Autodesk Inventor part; units mm, degrees
ref_plane "YZ Plane" through (0, 0, 0) normal (1, 0, 0) x (0, 1, 0)
ref_plane "XZ Plane" through (0, 0, 0) normal (0, 1, 0) x (-1, 0, 0)
ref_plane "XY Plane" through (0, 0, 0) normal (0, 0, 1) x (1, 0, 0)
sketch "Sketch1" plane through (0, 0, 0) normal (0, 0, 1) x (1, 0, 0)
  circle A0 centre (0, 0) radius 0.8
  circle A1 centre (0, 0) radius 0.4
  circle A2 centre (0, 0) radius 0.8
  circle A3 centre (0, 0) radius 1.5
  line L0 (0, 0) -> (-1.5, 0)
  line L1 (-0.8, 0) -> (-1.5, 0)
  line L2 (-2.1, 5) -> (-0.9, 5)
  line L3 (-0.9, 5) -> (-0.9, -5)
  line L4 (-0.9, -5) -> (-2.1, -5)
  line L5 (-2.1, -5) -> (-2.1, 5)
  line L6 (-2.1, 5) -> (-0.9, -5) construction
  line L7 (-0.9, 5) -> (-2.1, -5) construction
  point P0 (-0.9, -1.2)
  point P1 (-0.9, 1.2)
  dimension "d0" = 1.6
  dimension "d1" = 3
  dimension "d2" = 1.2
  dimension "d3" = 10
extrude "Extrusion1" add sketch "Sketch1" against normal blind 20 contours L3 A3 | L3 A3 L0 | L0 A3 L3 | A3 L3 L4 L5 L2
fillet "Fillet1" radius 0.5 2 edges at (-0.9, -1.2, -10) (-0.9, 1.2, -10)
chamfer "Chamfer1" distance 0.3 angle 45 2 edges at (-0.8, 0, -20) (-0.8, 0, 0)
sketch "Sketch2" plane through (-0.9, 5, 0) normal (1, 0, 0) x (0, 0, -1)
  line L0 (20, -3.0404) -> (0, -3.0404)
  line L1 (20, 0) -> (20, -3.0404)
  line L2 (0, 0) -> (20, 0)
  line L3 (0, -3.0404) -> (0, 0)
  line L4 (20, 0) -> (20, -3.0404)
  line L5 (20, 0) -> (20, -1)
  line L6 (20, -1) -> (16, -1)
  line L7 (16, -1) -> (10, -1)
  line L8 (10, -1) -> (4, -1)
  line L9 (4, -1) -> (0, -1)
  line L10 (0, -3.0404) -> (0, 0)
  circle A0 centre (16, -1) radius 0.6
  circle A1 centre (10, -1) radius 0.6
  circle A2 centre (4, -1) radius 0.6
  point P0 (0, -5)
  dimension "d10" = 1
  dimension "d11" = 4
  dimension "d12" = 6
  dimension "d13" = 6
  dimension "d14" = 1.2
  dimension "d15" = 1.2
  dimension "d16" = 1.2
extrude "Extrusion2" cut sketch "Sketch2" against normal blind 20 contours A0 L7 L6 | L6 L7 A0 | A2 L8 L9 | L9 L8 A2 | A1 L8 L7 | L7 L8 A1
sketch "Sketch3" plane through (-0.9, 5, 0) normal (1, 0, 0) x (0, 0, -1)
  circle A0 centre (4, -1) radius 0.6
  circle A1 centre (10, -1) radius 0.6
  circle A2 centre (16, -1) radius 0.6
  line L0 (20, -3.0404) -> (0, -3.0404)
  line L1 (20, 0) -> (20, -3.0404)
  line L2 (0, 0) -> (20, 0)
  line L3 (0, -3.0404) -> (0, 0)
  line L4 (17.5, -3) -> (17.5, 1)
  line L5 (17.5, 1) -> (14.5, 1)
  line L6 (14.5, 1) -> (14.5, -3)
  line L7 (14.5, -3) -> (17.5, -3)
  line L8 (17.5, -3) -> (14.5, 1) construction
  line L9 (17.5, 1) -> (14.5, -3) construction
  line L10 (11.5, 1) -> (11.5, -3)
  line L11 (11.5, -3) -> (8.5, -3)
  line L12 (8.5, -3) -> (8.5, 1)
  line L13 (8.5, 1) -> (11.5, 1)
  line L14 (11.5, 1) -> (8.5, -3) construction
  line L15 (11.5, -3) -> (8.5, 1) construction
  line L16 (5.5, 1) -> (5.5, -3)
  line L17 (5.5, -3) -> (2.5, -3)
  line L18 (2.5, -3) -> (2.5, 1)
  line L19 (2.5, 1) -> (5.5, 1)
  line L20 (5.5, 1) -> (2.5, -3) construction
  line L21 (5.5, -3) -> (2.5, 1) construction
  point P0 (0, -5)
  point P1 (2.5, 0)
  point P2 (5.5, 0)
  point P3 (8.5, 0)
  point P4 (11.5, 0)
  point P5 (14.5, 0)
  point P6 (17.5, 0)
  dimension "d19" = 4
  dimension "d20" = 3
  dimension "d21" = 4
  dimension "d22" = 3
  dimension "d23" = 4
  dimension "d24" = 3
extrude "Extrusion3" add sketch "Sketch3" against normal up to surface (1.2 mm away) contours L2 L6 L5 L4 | L18 L19 L16 L2 | L2 L12 L13 L10
ref_plane "Work Plane1" through (-2.1, 0, 0) normal (0, -1, 0) x (1, 0, 0)
mirror "Mirror1" about plane through (-2.1, 0, 0) normal (0, -1, 0) of "Extrusion2", "Extrusion3"
fillet "Fillet2" radius 0.5 12 edges at (-1.5, 5, -17.5) (-1.5, 5, -14.5) (-1.5, 5, -11.5) (-1.5, 5, -8.5) (-1.5, 5, -5.5) (-1.5, 5, -2.5) (-1.5, -5, -2.5) (-1.5, -5, -5.5) (-1.5, -5, -8.5) (-1.5, -5, -11.5) (-1.5, -5, -14.5) (-1.5, -5, -17.5)
chamfer "Chamfer2" distance 1 angle 45 4 edges at (-1.5, 5, -20) (-1.5, -5, -20) (-1.5, 5, 0) (-1.5, -5, 0)
properties part number "bl_tube_hn_1"
Check sheet for the modelled part. Datum: model origin and axes. Units: mm. A direction names the side the tool comes from. Give positions to 0.01 mm unless a question says otherwise; leave off trailing zeros. Order: outer loops, then holes, each group sorted by start corner. A loop starts at its lowest first (then second) coordinate and runs counter-clockwise, first axis right, second up. Notation, with made-up numbers: M 30,-8 L 52,-8 A9 ccw 52,-2 Z; hole C 58,13 d3. An arc over 180 degrees is marked long. Answer in a Markdown table with one row per item. Add a question column.
Q1. Sectioned sample at B-B, the plane z = -18.5. Record the boundary of the cut face in (x, y).
Q2. Release check for a two-part mould opening along Z. For faces 5 (the conical face through (-0.02, -0.92, -0.18)), 6 (the conical face through (0.02, -0.92, -19.82)), 7 (the flat face through (-1.5, 5, -13)) record: released by +Z, released by -Z, zero draft, split by the parting line, or undercut.
Q3. Thickness scan on L1, parallel to Y at x = -1.8, z = -10; L2, parallel to X at y = 2, z = -13; L3, parallel to X at y = 0.5, z = -12. Record the ranges inside material, lowest first.
Q4. Sectioned sample at C-C, the plane x = -1.6. Count the separate pieces of the cut face and the enclosed holes in it, and give its area (3 significant figures).
Q5. Sectioned sample at D-D, the plane y = 2.25. Record the boundary of the cut face in (x, z), and give its area (3 significant figures).
Q6. Sectioned sample at A-A, the plane z = -4. Record the boundary of the cut face in (x, y).
Q7. Access from +Z, -Z, +X, -X, +Y, -Y to the whole of each face (thin tool, end or side, straight path). Record for faces 1 (the flat face through (-0.9, -3, -10)), 2 (the cylindrical face through (-1.5, 4, -3.4)), 3 (the flat face through (-1.5, -5, -18.5)), 4 (the flat face through (-0.9, 3, -10)).
Q8. Gauge pin test, flat ends, axial feed: pin 1 Ø2 at (y, z) = (4.5, -7.5) entering from +X; pin 2 Ø0.6 at (x, y) = (-1.5, 6) entering from +Z; pin 3 Ø0.6 at (x, y) = (-1.5, 5.5) entering from -Z. Record the tip position at first contact, or that the pin passes through.
Verdict:
| question | item | result |
|---|---|---|
| 1 | outline | M -2.1,-5 L -0.9,-5 L -0.9,-1.96 A0.5 cw -0.3,-1.47 A1.5 ccw long -0.3,1.47 A0.5 cw -0.9,1.96 L -0.9,5 L -2.1,5 Z; hole C 0,0 d1.6 |
| 2 | face 5 | released by +Z |
| 2 | face 6 | released by -Z |
| 2 | face 7 | undercut |
| 3 | L1 | -6 to -4.6, -3.4 to 3.4, 4.6 to 6 |
| 3 | L2 | -2.1 to -0.9 |
| 3 | L3 | -2.1 to -0.62, 0.62 to 1.41 |
| 4 | separate pieces | 1 |
| 4 | enclosed holes | 6 |
| 4 | area | 210 mm² |
| 5 | outline | M -2.1,-20 L -0.9,-20 L -0.9,0 L -2.1,0 Z |
| 5 | area | 24.0 mm² |
| 6 | outline | M -2.1,-6 L -0.9,-6 L -0.9,-4.6 L -2.1,-4.6 Z; M -2.1,-3.4 L -0.9,-3.4 L -0.9,-1.96 A0.5 cw -0.3,-1.47 A1.5 ccw long -0.3,1.47 A0.5 cw -0.9,1.96 L -0.9,3.4 L -2.1,3.4 Z; M -2.1,4.6 L -0.9,4.6 L -0.9,6 L -2.1,6 Z; hole C 0,0 d1.6 |
| 7 | face 1 | +Z, -Z, +X, -Y |
| 7 | face 2 | +X, -X |
| 7 | face 3 | -Z, +X, -X, -Y |
| 7 | face 4 | +Z, -Z, +X, +Y |
| 8 | pin 1 | x = -0.9 |
| 8 | pin 2 | z = -2.5 |
| 8 | pin 3 | z = -17.6 |
